Geometry: final body of the model. Coordinates: model frame, mm. Give positions to 0.01 mm unless a question says otherwise; leave off trailing zeros. Loops run counter-clockwise (first coordinate to the right, second up) from the corner with the lowest first, then second, coordinate; pieces in that order, holes last.
from build123d import *

# Parameters (mm, degrees)
SKETCH1_W           = 20
SKETCH1_H           = 5
SKETCH1_W_2         = 5
SKETCH1_H_2         = 30
BOSS_EXTRUDE1_DEPTH = 5


with BuildPart() as part:
    # Sketch1 → Boss-Extrude1 (new body)
    with BuildSketch(Plane.XY):
        Polygon((85, -102.314739042), (85, -4.053866158), (34, 64.685260958), (-65, 64.685260958), (-153, -37.314739042), (-153, -102.314739042), (-65, -176.314739042), (45, -176.314739042), align=None)
        with Locations((-55, -143.814739042)):
            Rectangle(SKETCH1_W, SKETCH1_H, mode=Mode.SUBTRACT)
        with Locations((-55, -121.814739042)):
            Rectangle(SKETCH1_W, SKETCH1_H, mode=Mode.SUBTRACT)
        with Locations((-103, -61.814739042)):
            Rectangle(SKETCH1_W, SKETCH1_H, mode=Mode.SUBTRACT)
        with Locations((-40, -99.814739042)):
            Rectangle(SKETCH1_W, SKETCH1_H, mode=Mode.SUBTRACT)
        with Locations((-57.5, -77.314739042)):
            Rectangle(SKETCH1_W_2, SKETCH1_H_2, mode=Mode.SUBTRACT)
        with Locations((24, -143.814739042)):
            Rectangle(SKETCH1_W, SKETCH1_H, mode=Mode.SUBTRACT)
        with Locations((24, -121.622499161)):
            Rectangle(SKETCH1_W, SKETCH1_H, mode=Mode.SUBTRACT)
        with Locations((0, -99.814739042)):
            Rectangle(SKETCH1_W, SKETCH1_H, mode=Mode.SUBTRACT)
        with Locations((-24, -61.814739042)):
            Rectangle(SKETCH1_W, SKETCH1_H, mode=Mode.SUBTRACT)
        with Locations((17.5, -77.314739042)):
            Rectangle(SKETCH1_W_2, SKETCH1_H_2, mode=Mode.SUBTRACT)
        with Locations((55, -61.814739042)):
            Rectangle(SKETCH1_W, SKETCH1_H, mode=Mode.SUBTRACT)
        with Locations((-55, -39.814739042)):
            Rectangle(SKETCH1_W, SKETCH1_H, mode=Mode.SUBTRACT)
        with Locations((-57.5, -7.314739042)):
            Rectangle(SKETCH1_W_2, SKETCH1_H_2, mode=Mode.SUBTRACT)
        Polygon((-65, 22.685260958), (-45, 22.685260958), (-45, 17.685260958), (-30, 17.685260958), (-30, 12.685260958), (-50, 12.685260958), (-50, 17.685260958), (-65, 17.685260958), align=None, mode=Mode.SUBTRACT)
        with Locations((-55, 42.185260958)):
            Rectangle(SKETCH1_W, SKETCH1_H, mode=Mode.SUBTRACT)
        with Locations((24, -39.814739042)):
            Rectangle(SKETCH1_W, SKETCH1_H, mode=Mode.SUBTRACT)
        with Locations((17.5, -7.314739042)):
            Rectangle(SKETCH1_W_2, SKETCH1_H_2, mode=Mode.SUBTRACT)
        with Locations((-6, 15.185260958)):
            Rectangle(SKETCH1_W, SKETCH1_H, mode=Mode.SUBTRACT)
        with Locations((24, 20.185260958)):
            Rectangle(SKETCH1_W, SKETCH1_H, mode=Mode.SUBTRACT)
        with Locations((24, 42.185260958)):
            Rectangle(SKETCH1_W, SKETCH1_H, mode=Mode.SUBTRACT)
    extrude(amount=BOSS_EXTRUDE1_DEPTH)


solid = part.part
Item 1: Pin query (flat end, axial travel): pin 1 (1.5 mm diameter, centred on x = 56, z = 2.5, fed in from +Y); pin 2 (3 mm diameter, centred on x = 6, y = -61.5, fed in from -Z); pin 3 (1 mm diameter, centred on x = -78.5, z = 2.5, fed in from -Y). Return the tip coordinate at first contact, or that it passes through.
Values follow:
pin 1: stops at y = 36.04
pin 2: stops at z = 0
pin 3: stops at y = -165.38
Item 2: Ray query, probe 1 along X at (y, z) = (-71, 2.2); probe 2 along Y at (x, z) = (32, 2.2); probe 3 along Y at (x, z) = (-61, 0.8). Return the intervals inside material, ascending.
Values follow:
probe 1: x = -153 to -60, -55 to 15, 20 to 85
probe 2: y = -176.31 to -146.31, -141.31 to -124.12, -119.12 to -42.31, -37.31 to 17.69, 22.69 to 39.69, 44.69 to 64.69
probe 3: y = -176.31 to -146.31, -141.31 to -124.31, -119.31 to -42.31, -37.31 to 17.69, 22.69 to 39.69, 44.69 to 64.69
Item 3: Section query B-B on x = -108. Return loops of the section in (y, z), plus the area to 3 significant figures.
Values follow:
outline: (-140.16, 0) - (-64.31, 0) - (-64.31, 5) - (-140.16, 5) - close; (-59.31, 0) - (14.84, 0) - (14.84, 5) - (-59.31, 5) - close
area: 750 mm2
Item 4: Section query D-D on y = -112.5. Return loops of the section in (x, z).
Values follow:
outline: (-140.89, 0) - (79.49, 0) - (79.49, 5) - (-140.89, 5) - close
Item 5: Section query A-A on x = -40. Return loops of the section in (y, z).
Values follow:
outline: (-176.31, 0) - (-102.31, 0) - (-102.31, 5) - (-176.31, 5) - close; (-97.31, 0) - (12.69, 0) - (12.69, 5) - (-97.31, 5) - close; (17.69, 0) - (64.69, 0) - (64.69, 5) - (17.69, 5) - close
Item 6: Section query C-C on z = 2.2. Give the number of separate pieces and of enclosed holes in the cut face, plus the area to 3 significant figures.
Values follow:
separate pieces: 1
enclosed holes: 20
area: 44,100 mm2
